The model under review builds one solid part; all positions refer to its coordinate system, in mm. Face numbers are marked on the shaded views. A direction names the side the tool comes from. Round coordinates to 2 decimals unless told otherwise and drop trailing zeros. Write each loop counter-clockwise with the first axis right and the second up, starting at its lowest first coordinate (ties: lowest second). Pieces come first, ordered by that corner, then holes. Notation, with made-up numbers: (47, 35.5) - (59, 35.5) arc R24 ccw to (59, 66.5) - close; hole circle Ø5 at (11, 62). An arc over 180 degrees is marked (long way). Return JSON: item names as keys, results as strings.
from build123d import *

# Parameters (mm, degrees)
BOSS_EXTRUDE1_DEPTH = 1900
SKETCH2_R           = 300
CUT_EXTRUDE1_DEPTH  = 2232.591360442
SKETCH4_W           = 250
SKETCH4_H           = 100
CUT_EXTRUDE3_DEPTH  = 550
SHELL1_START        = 320
SHELL1_DEPTH        = 1560
SHELL1_START_2      = 20
SHELL1_2_DEPTH      = 300
SHELL1_3_DEPTH      = 10


# Read off the part's stored shape, not the designer's step: Shell1
with BuildPart() as part:
    # Sketch1 → Boss-Extrude1 (new body)
    with BuildSketch(Plane.XY):
        with BuildLine():
            Line((931.575680567, 120), (1100, 120))
            Line((1100, 120), (1100, 0))
            Line((1100, 0), (0, 0))
            Line((0, 0), (0, 120))
            Line((0, 120), (168.424319433, 120))
            ThreePointArc((168.424319433, 120), (550, 400), (931.575680567, 120))
        make_face()
    extrude(amount=BOSS_EXTRUDE1_DEPTH)

    # Sketch2 → Cut-Extrude1 (cut, through all)
    with BuildSketch(Plane.XY.offset(1900)):
        with Locations((550, 0)):
            Circle(SKETCH2_R)
    extrude(amount=-CUT_EXTRUDE1_DEPTH, mode=Mode.SUBTRACT)

    # Sketch4 → Cut-Extrude3 (cut)
    with BuildSketch(Plane(origin=(1100, 0, 0), x_dir=(0, 0, -1), z_dir=(1, 0, 0))):
        with Locations((-175, 50)):
            Rectangle(SKETCH4_W, SKETCH4_H)
    extrude(amount=-CUT_EXTRUDE3_DEPTH, mode=Mode.SUBTRACT)

    # Shell1 outline → Shell1 (cut)
    with BuildSketch(Plane.XY.offset(SHELL1_START)):
        with BuildLine():
            ThreePointArc((916.606055596, 100), (550, 380), (183.393944404, 100))
            Line((183.393944404, 100), (20, 100))
            Line((20, 100), (20, 0))
            Line((20, 0), (250, 0))
            ThreePointArc((250, 0), (550, 300), (850, 0))
            Line((850, 0), (1080, 0))
            Line((1080, 0), (1080, 100))
            Line((1080, 100), (916.606055596, 100))
        make_face()
    extrude(amount=SHELL1_DEPTH, mode=Mode.SUBTRACT)

    # Shell1 2 outline → Shell1 2 (cut)
    with BuildSketch(Plane.XY.offset(SHELL1_START_2)):
        with BuildLine():
            Line((824.954541697, 120), (910.555127546, 120))
            ThreePointArc((910.555127546, 120), (539.552347988, 379.856349911), (183.393944404, 100))
            Line((183.393944404, 100), (20, 100))
            Line((20, 100), (20, 0))
            Line((20, 0), (250, 0))
            ThreePointArc((250, 0), (488.707106893, 293.671893879), (824.954541697, 120))
        make_face()
    extrude(amount=SHELL1_2_DEPTH, mode=Mode.SUBTRACT)

    # Shell1 3 outline → Shell1 3 (cut)
    with BuildSketch(Plane.XY.offset(SHELL1_START_2)):
        with BuildLine():
            ThreePointArc((916.606055596, 100), (913.718086665, 110.041598646), (910.555127546, 120))
            Line((910.555127546, 120), (824.954541697, 120))
            ThreePointArc((824.954541697, 120), (843.671893879, 61.292893107), (850, 0))
            Line((850, 0), (1080, 0))
            Line((1080, 0), (1080, 100))
            Line((1080, 100), (916.606055596, 100))
        make_face()
    extrude(amount=SHELL1_3_DEPTH, mode=Mode.SUBTRACT)


solid = part.part
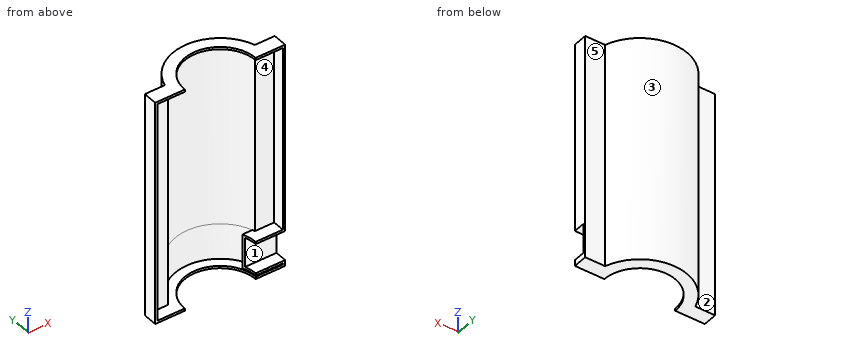
(1) Add section C-C (x = 550). Write out the cut boundary in (y, z).
Filled in:
{"outline": "(300, 0) - (400, 0) - (400, 1900) - (300, 1900) - (300, 1880) - (380, 1880) - (380, 20) - (300, 20) - close"}
(2) Wall thickness on line 1 (Z direction, x = 878, y = 27.5); line 2 (X direction, y = 336.5, z = 1637); line 3 (X direction, y = 270.5, z = 1685.5): over which ranges is each line inside the solid? List them lowest first.
Filled in:
{"line 1": "z = 0 to 20, 30 to 50, 300 to 320, 1880 to 1900", "line 2": "x = 333.74 to 373.46, 726.54 to 766.26", "line 3": "x = 255.33 to 283.11, 816.89 to 844.67"}
(3) Add section A-A (y = 259). Write out the cut boundary in (x, z), plus the area to 3 significant figures.
Filled in:
{"outline": "(245.17, 0) - (398.61, 0) - (398.61, 20) - (271.94, 20) - (271.94, 1880) - (398.61, 1880) - (398.61, 1900) - (245.17, 1900) - close; (701.39, 0) - (854.83, 0) - (854.83, 1900) - (701.39, 1900) - (701.39, 1880) - (828.06, 1880) - (828.06, 20) - (701.39, 20) - close", "area": "112,000 mm2"}
(4) Mouldability with a two-part tool opening along Z and no side actions: class the marked faces 1 and 2 as released by +Z, released by -Z, zero draft, split by the parting line, or undercut.
Filled in:
{"face 1": "undercut", "face 2": "zero draft"}
(5) Add section D-D (x = 689.5). Write out the cut boundary in (y, z).
Filled in:
{"outline": "(265.59, 0) - (374.89, 0) - (374.89, 1900) - (265.59, 1900) - (265.59, 1880) - (353.47, 1880) - (353.47, 20) - (265.59, 20) - close"}
(6) For the marked faces 3, 4 and 5, list the 3-axis set-ups (+Z, -Z, +X, -X, +Y, -Y) from which the entire face can be reached by the end or side of a thin tool; tool diameter is ignored.
Filled in:
{"face 3": "+Z, -Z, +Y", "face 4": "-Y", "face 5": "+Z, -Z, +X, +Y"}
(7) Add section B-B (z = 880.5). Write out the cut boundary in (x, y).
Filled in:
{"outline": "(0, 0) - (20, 0) - (20, 100) - (183.39, 100) arc R380 cw to (916.61, 100) - (1080, 100) - (1080, 0) - (1100, 0) - (1100, 120) - (931.58, 120) arc R400 ccw to (168.42, 120) - (0, 120) - close"}
(8) Clearance check with flat-ended pins moving along their axes: pin 1 Ø4 at (y, z) = (267.5, 416) entering from +X; pin 2 Ø12 at (x, z) = (204, 677.5) entering from +Y; pin 3 Ø1.5 at (x, z) = (660, 263.5) entering from -Y. State where each tip first meets the part, or that it passes through.
Filled in:
{"pin 1": "stops at x = 849.18", "pin 2": "stops at y = 210.71", "pin 3": "stops at y = 363.5"}
